Can you work these out from the drawing? Everything is in mm from the part's minimum corner. A direction names the side the tool comes from. Round coordinates to 2 decimals unless told otherwise and drop trailing zeros. Order: outer loops, then holes, each group sorted by start corner. A loop starts at its lowest first (then second) coordinate and runs counter-clockwise, first axis right, second up. Notation, with made-up numbers: (-1, -4) -> (37, -4) arc R19 cw to (37, 32) -> close; hole circle Ø1 at (2.5, -31). An arc over 180 degrees is marked (long way). One line per item, written item: value.
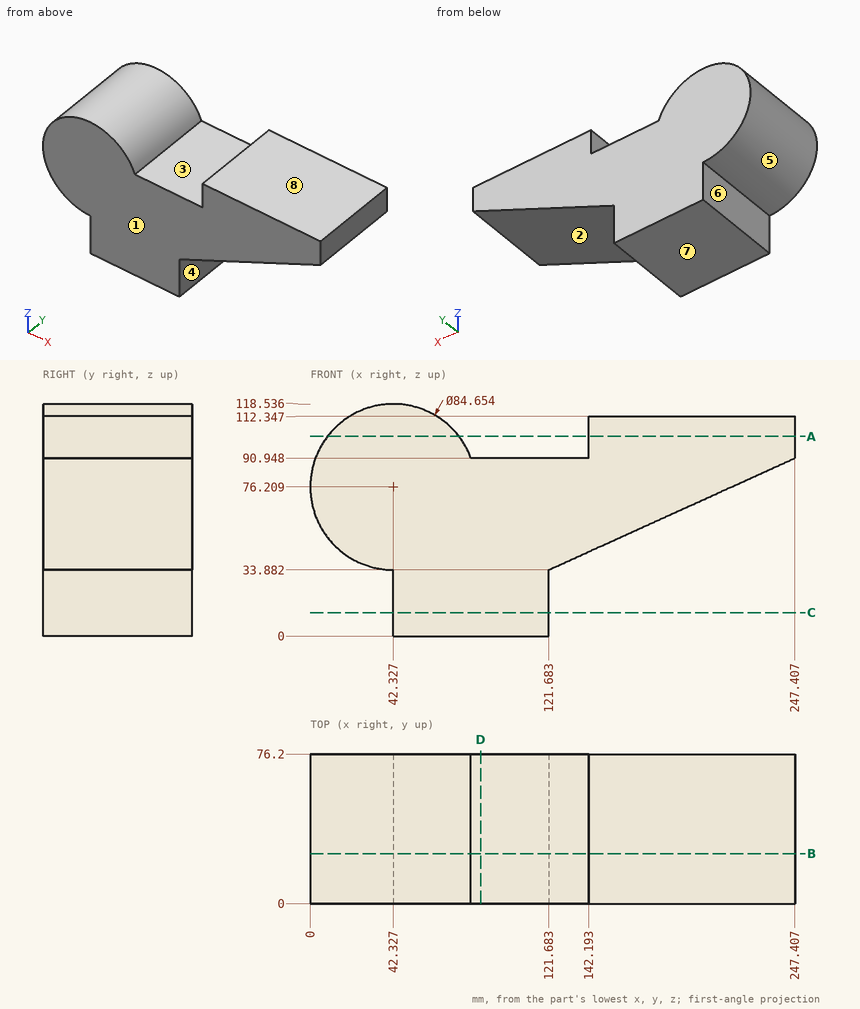
Q1. For P1, Ø17, axis at y = 24.5, z = 20, coming from the +X side; P2, Ø6, axis at y = 38.5, z = 102, coming from the -X side; P3, Ø10.5, axis at y = 38, z = 102, coming from the -X side, each with a flat end and sliding along its axis, tell me the tip position at first contact or that it passes through.
Answers:
P1: x = 121.68
P2: x = 6.66
P3: x = 5.32
Q2. Which directions (+Z, -Z, +X, -X, +Y, -Y) give clear straight access to the entire face, cutting with the end or side of a thin tool? Please do the marked faces 4, 5, 6, 7 and 8.
Answers:
face 4: -Z, +X, +Y, -Y
face 5: +Y, -Y
face 6: -Z, -X, +Y, -Y
face 7: -Z, +X, -X, +Y, -Y
face 8: +Z, +X, +Y, -Y
Q3. I want a section at A-A on z = 102. Write out the boundary of the cut face in (x, y) (1 decimal).
Answers:
outline: (8.8, 0) -> (75.9, 0) -> (75.9, 76.2) -> (8.8, 76.2) -> close; (142.2, 0) -> (247.4, 0) -> (247.4, 76.2) -> (142.2, 76.2) -> close
Q4. I want a section at C-C on z = 12. Write out the boundary of the cut face in (x, y), then the cut area to 3 significant figures.
Answers:
outline: (42.33, 0) -> (121.68, 0) -> (121.68, 76.2) -> (42.33, 76.2) -> close
area: 6,050 mm2
Q5. I want a section at B-B on y = 25.5. Write out the boundary of the cut face in (x, z) (1 decimal).
Answers:
outline: (42.3, 0) -> (121.7, 0) -> (121.7, 33.9) -> (247.4, 90.9) -> (247.4, 112.3) -> (142.2, 112.3) -> (142.2, 90.9) -> (82, 90.9) arc R42.3 ccw (long way) to (42.3, 33.9) -> close
Q6. I need wall thicknesses on line 1 along X through (y, z) = (51, 18.5); line 2 along X through (y, z) = (4, 108) (1 decimal); line 3 along X through (y, z) = (11.5, 99.5) (1 decimal). Which ranges of each line are inside material? Lowest first, please.
Answers:
line 1: 42.33 to 121.68
line 2: 14.4 to 70.3, 142.2 to 247.4
line 3: 7 to 77.7, 142.2 to 247.4
Q7. I want a section at D-D on x = 87. Write out the boundary of the cut face in (y, z), then the cut area to 3 significant figures.
Answers:
outline: (0, 0) -> (76.2, 0) -> (76.2, 90.95) -> (0, 90.95) -> close
area: 6,930 mm2
Q8. If we mould it in two halves opening along X, with no side actions, what happens to the marked faces 1, 2 and 3? For each: pulls with the +X half, pulls with the -X half, needs draft (parallel to the pull), parting line crosses it, or undercut.
Answers:
face 1: needs draft
face 2: pulls with the +X half
face 3: undercut
